```python
from build123d import *

# Parameters (mm, degrees)
F1_DEPTH      = 127
F1_DEPTH_BACK = 127
F2_R          = 3.175
F3_DEPTH      = 25.401
F5_D          = 7.8994
F5_DEPTH      = 12.7


with BuildPart() as f1:
    # F0 (on Right) → F1 (new body, two sides)
    with BuildSketch(Plane.YZ) as f1_sk:
        Polygon((-38.1, -0.9017), (36.2966, -0.9017), (36.2966, -24.4983), (38.1, -24.4983), (38.1, -0.9017), (38.1, 0.9017), (-38.1, 0.9017), align=None)
    extrude(amount=F1_DEPTH)
    extrude(f1_sk.sketch, amount=-F1_DEPTH_BACK)

    # F2 (on face) → F3 (cut, through all)
    with BuildSketch(Plane.XY.offset(0.9017)):
        with Locations((-25.4, 5.08)):
            Circle(F2_R)
        with Locations((25.4, 5.08)):
            Circle(F2_R)
    extrude(amount=-F3_DEPTH, mode=Mode.SUBTRACT)

    # F5
    with Locations(Plane(origin=(0, 38.1, 0), x_dir=(-1, 0, 0), z_dir=(0, 1, 0))):
        with Locations((-63.5381, -15.5321), (63.5381, -15.5321)):
            Hole(F5_D / 2, depth=F5_DEPTH)


solid = f1.part
```
Part model, mm, in its own coordinate system. A direction names the side the tool comes from. Round coordinates to 2 decimals unless told otherwise and drop trailing zeros. Loops run counter-clockwise (first coordinate to the right, second up) from the corner with the lowest first, then second, coordinate; pieces in that order, holes last. Notation, with made-up numbers: (27.5, 43.25) -> (63.5, 43.25) arc R20 ccw to (63.5, 53.25) -> close; hole circle Ø8 at (58, -1.75). An arc over 180 degrees is marked (long way). Use a Markdown table: item, result.
1) Tool access for faces 1 (the cylindrical face through (-22.47, 3.86, 0.01)), 2 (the flat face through (2, -1, -0.902)): list every direction of +Z, -Z, +X, -X, +Y, -Y with a clear straight run to the whole face (end or side of a thin tool).
The answers:
| item | result |
|---|---|
| face 1 | +Z, -Z |
| face 2 | -Z, +X, -X, -Y |
2) Cut at A-A, the plane y = 5.08. List the corners of the cut face in (x, z) (3 decimals), and give its area (3 significant figures).
The answers:
| item | result |
|---|---|
| outline | (-127, -0.902) -> (-28.575, -0.902) -> (-28.575, 0.902) -> (-127, 0.902) -> close; (-22.225, -0.902) -> (22.225, -0.902) -> (22.225, 0.902) -> (-22.225, 0.902) -> close; (28.575, -0.902) -> (127, -0.902) -> (127, 0.902) -> (28.575, 0.902) -> close |
| area | 435 mm2 |
3) Probe line 1 (Z direction, x = 45, y = -9); line 2 (Y direction, x = 14, z = -11); line 3 (Y direction, x = 25.4, z = -0.5) (3 decimals). List the from-to ranges inside material, lowest first. Write a range as [from, to].
The answers:
| item | result |
|---|---|
| line 1 | z = [-0.9, 0.9] |
| line 2 | y = [36.3, 38.1] |
| line 3 | y = [-38.1, 1.905], [8.255, 38.1] |
4) Cut at C-C, the plane y = 18.5. List the corners of the cut face in (x, z), and give its area (3 significant figures).
The answers:
| item | result |
|---|---|
| outline | (-127, -0.9) -> (127, -0.9) -> (127, 0.9) -> (-127, 0.9) -> close |
| area | 458 mm2 |
5) Cut at B-B, the plane x = 25.4. List the corners of the cut face in (y, z) (3 decimals), and give its area (3 significant figures).
The answers:
| item | result |
|---|---|
| outline | (-38.1, -0.902) -> (1.905, -0.902) -> (1.905, 0.902) -> (-38.1, 0.902) -> close; (8.255, -0.902) -> (36.297, -0.902) -> (36.297, -24.498) -> (38.1, -24.498) -> (38.1, 0.902) -> (8.255, 0.902) -> close |
| area | 169 mm2 |
6) Pull direction X, two halves, no side cores. Call faces 3 (the cylindrical face through (28.33, 3.86, 0.01)), 4 (the flat face through (127, 11, 0)), 5 (the flat face through (2, 36.297, -13)): pulls with the +X half, pulls with the -X half, needs draft (parallel to the pull), parting line crosses it, or undercut.
The answers:
| item | result |
|---|---|
| face 3 | undercut |
| face 4 | pulls with the +X half |
| face 5 | needs draft |
7) Drop flat-ended pins along their axis: pin 1 Ø6.5 at (x, z) = (-63.54, -15.53) entering from -Y; pin 2 Ø8 at (x, y) = (77, -15) entering from -Z; pin 3 Ø4 at (x, z) = (54.5, -12) entering from -Y. Give the stop position or say it passes through.
The answers:
| item | result |
|---|---|
| pin 1 | passes through |
| pin 2 | stops at z = -0.9 |
| pin 3 | stops at y = 36.3 |
